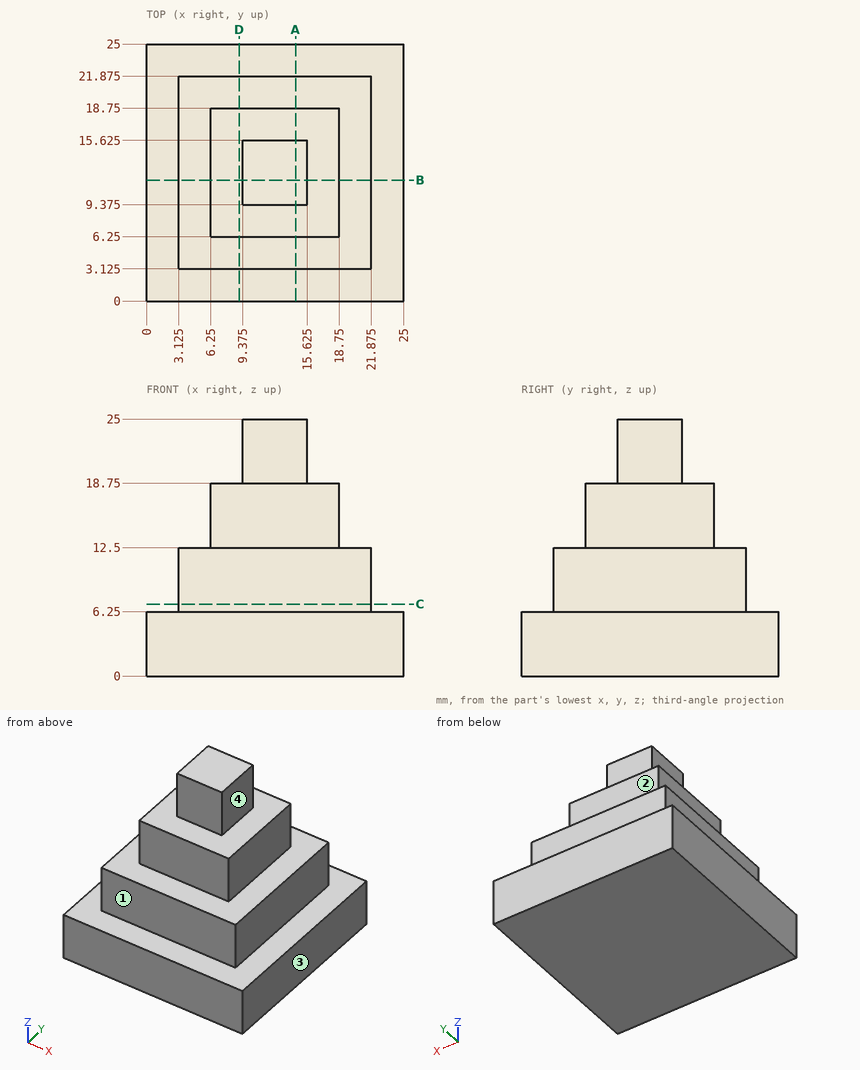
Print and shaded views of the part. All mm, measured from the part's lowest x, y and z. A direction names the side the tool comes from. Give positions to 0.01 mm unless a question says otherwise; leave off trailing zeros. Loops run counter-clockwise (first coordinate to the right, second up) from the corner with the lowest first, then second, coordinate; pieces in that order, holes last. Notation, with made-up numbers: (80, 16) - (131, 16) arc R25 cw to (131, 40) - close; hole circle Ø2 at (39, 56). An arc over 180 degrees is marked (long way). One line per item, written item: value. Start each with the question number.
1. Slice it at C-C (z = 7). List the corners of the cut face in (x, y) (3 decimals).
2. Slice it at D-D (x = 9). List the corners of the cut face in (y, z) (3 decimals).
3. Slice it at A-A (x = 14.5). List the corners of the cut face in (y, z) (3 decimals).
4. Which spindle directions (+Z, -Z, +X, -X, +Y, -Y) get a long thin tool onto all of the face, cutting with end or side? Do the marked faces 1, 2, 3 and 4. Say none if no direction does.
5. Pin check, flat tips, straight feed: pin 1 (5 mm diameter, centred on y = 14, z = 21.5, fed in from -X) (3 decimals); pin 2 (5 mm diameter, centred on x = 13, z = 15.5, fed in from +Y); pin 3 (5 mm diameter, centred on y = 13.5, z = 16.5, fed in from -X). Stop position of each tip, or through.
6. Probe L1, parallel to Y at x = 17.5, z = 8.5 (3 decimals); L2, parallel to Z at x = 16, y = 3; L3, parallel to Z at x = 5.5, y = 9.5. List the from-to ranges inside material, lowest first. Write a range as from..to.
Solution:
1. outline: (3.125, 3.125) - (21.875, 3.125) - (21.875, 21.875) - (3.125, 21.875) - close
2. outline: (0, 0) - (25, 0) - (25, 6.25) - (21.875, 6.25) - (21.875, 12.5) - (18.75, 12.5) - (18.75, 18.75) - (6.25, 18.75) - (6.25, 12.5) - (3.125, 12.5) - (3.125, 6.25) - (0, 6.25) - close
3. outline: (0, 0) - (25, 0) - (25, 6.25) - (21.875, 6.25) - (21.875, 12.5) - (18.75, 12.5) - (18.75, 18.75) - (15.625, 18.75) - (15.625, 25) - (9.375, 25) - (9.375, 18.75) - (6.25, 18.75) - (6.25, 12.5) - (3.125, 12.5) - (3.125, 6.25) - (0, 6.25) - close
4. face 1: +Z, +X, -X, -Y
4. face 2: +Z, +X, -X, +Y
4. face 3: +Z, -Z, +X, +Y, -Y
4. face 4: +Z, +X, +Y, -Y
5. pin 1: stops at x = 9.375
5. pin 2: stops at y = 18.75
5. pin 3: stops at x = 6.25
6. L1: y = 3.125..21.875
6. L2: z = 0..6.25
6. L3: z = 0..12.5
